```python
from build123d import *

# Parameters (mm, degrees)
SKETCH_1_R      = 1.45
EXTRUDE_1_DEPTH = 3
FILLET_1_R      = 10


with BuildPart() as part:
    # 草图1 → 凸台-拉伸1 (new body)
    with BuildSketch(Plane.XY):
        with BuildLine():
            Line((0, 0), (25, 0))
            ThreePointArc((25, 0), (56.497933188, -33.723935553), (69.5, -78))
            Line((69.5, -78), (77.5, -78))
            ThreePointArc((77.5, -78), (62.96989722, -27.008015863), (25, 10))
            Line((25, 10), (0, 10))
            ThreePointArc((0, 10), (-37.96989722, -27.008015863), (-52.5, -78))
            Line((-52.5, -78), (-44.5, -78))
            ThreePointArc((-44.5, -78), (-31.497933188, -33.723935553), (0, 0))
        make_face()
        with Locations((5, 5)):
            Circle(SKETCH_1_R, mode=Mode.SUBTRACT)
        with Locations((20, 5)):
            Circle(SKETCH_1_R, mode=Mode.SUBTRACT)
    extrude(amount=EXTRUDE_1_DEPTH)

    # 圆角1
    fillet_1_edges = [part.edges().sort_by_distance(p)[0] for p in [
        (0, 10, 1.5),
        (25, 10, 1.5),
        (25, 0, 1.5),
        (0, 0, 1.5),
    ]]
    fillet(fillet_1_edges, radius=FILLET_1_R)


solid = part.part
```
Source: CAD feature listing. Evaluate the final solid. Frame: model axes, mm. A direction names the side the tool comes from. Round coordinates to 2 decimals unless told otherwise and drop trailing zeros. Loops run counter-clockwise (first coordinate to the right, second up) from the corner with the lowest first, then second, coordinate; pieces in that order, holes last.
(1) Section query A-A (x = 20). Output: boundary loops of the cut face in (y, z), and give its area (3 significant figures).
From the geometry:
outline: (0, 0) - (3.55, 0) - (3.55, 3) - (0, 3) - close; (6.45, 0) - (10, 0) - (10, 3) - (6.45, 3) - close
area: 21.3 mm2
(2) Pull-direction query (X, two-part tool) for faces 3 (the cylindrical face through (25.01, 9.63, 1.52)), 4 (the cylindrical face through (-0.01, 9.63, 1.52)), 5 (the flat face through (12, 0, 1)); classes: +X half, -X half, draft (parallel to the pull), parting line (faces both ways), or undercut.
From the geometry:
face 3: +X half
face 4: -X half
face 5: undercut
(3) Contact query for flat-ended pins moving along their axis: pin 1 Ø2.5 at (x, y) = (20, 5) entering from +Z; pin 2 Ø3.5 at (x, y) = (5, 5) entering from -Z; pin 3 Ø1 at (y, z) = (-57, 1) entering from +X. Output: stop coordinate, or through.
From the geometry:
pin 1: passes through
pin 2: stops at z = 0
pin 3: stops at x = 75.08
(4) Access query for faces 1 (the cylindrical face through (56.99, -34.6, 1.48)), 2 (the flat face through (-2, -1, 3)). Directions: +Z, -Z, +X, -X, +Y, -Y. A direction counts if a zero-diameter tool reaches every point of the face in a straight line with its end or side. Return the directions, or none.
From the geometry:
face 1: +Z, -Z, -Y
face 2: +Z, +X, -X, +Y, -Y
(5) Section query D-D (x = 65). Output: boundary loops of the cut face in (y, z).
From the geometry:
outline: (-53.17, 0) - (-30.57, 0) - (-30.57, 3) - (-53.17, 3) - close
(6) Section query B-B (z = 0.45). Output: boundary loops of the cut face in (x, y).
From the geometry:
outline: (-52.5, -78) - (-44.5, -78) arc R100 cw to (-2.7, -1.86) arc R10 cw to (3.11, 0) - (21.89, 0) arc R10 cw to (27.7, -1.86) arc R100 cw to (69.5, -78) - (77.5, -78) arc R103 ccw to (27.45, 8.58) arc R10 ccw to (22.31, 10) - (2.69, 10) arc R10 ccw to (-2.45, 8.58) arc R103 ccw to start; hole circle Ø2.9 at (5, 5); hole circle Ø2.9 at (20, 5)
(7) Material intervals for probe 1 along Y at (x, z) = (20, 1); probe 2 along X at (y, z) = (6, 1.95); probe 3 along X at (y, z) = (4.5, 1.45), sorted ascending.
From the geometry:
probe 1: y = 0 to 3.55, 6.45 to 10
probe 2: x = -6.53 to 3.95, 6.05 to 18.95, 21.05 to 31.53
probe 3: x = -8.73 to 3.64, 6.36 to 18.64, 21.36 to 33.73
(8) Section query C-C (y = -23.5). Output: boundary loops of the cut face in (x, z).
From the geometry:
outline: (-35.78, 0) - (-24.81, 0) - (-24.81, 3) - (-35.78, 3) - close; (49.81, 0) - (60.78, 0) - (60.78, 3) - (49.81, 3) - close
